```python
from build123d import *

# Parameters (mm, degrees)
HOLE_WIZARD_M3_1_D = 2.5


with BuildPart() as part:
    # 草图1 → 旋转1 (revolve)
    with BuildSketch(Plane.XY, mode=Mode.PRIVATE) as revolve_1_sk:
        Polygon((70, 0), (76.75, 0), (76.75, 3), (75, 3), (75, 11), (70, 11), align=None)
    revolve(revolve_1_sk.sketch.rotate(Axis((0, 51.694672702, 0), (0, -1, 0)), 90), axis=Axis((0, 51.694672702, 0), (0, -1, 0)))

    # M3 螺纹孔1 (through all)
    with Locations(Plane(origin=(0, 11, 0), x_dir=(1, 0, 0), z_dir=(0, 1, 0))):
        with Locations((-51.265241636, 51.265241636), (0, 72.5), (51.265241636, 51.265241636), (72.5, 0), (51.265241636, -51.265241636), (0, -72.5), (-51.265241636, -51.265241636), (-72.5, 0)):
            Hole(HOLE_WIZARD_M3_1_D / 2)


solid = part.part
```
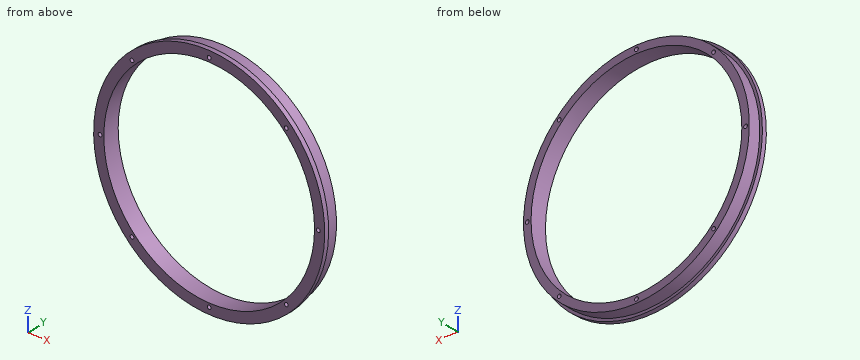
Part model, mm, in its own coordinate system. Coordinates: 2 decimals unless noted, no trailing zeros. Loops run counter-clockwise (first coordinate to the right, second up) from the corner with the lowest first, then second, coordinate; pieces in that order, holes last. Notation, with made-up numbers: (33.25, 87.25) - (52.25, 87.25) arc R24 cw to (52.25, 98.25) - close; hole circle Ø3 at (33, 82). An arc over 180 degrees is marked (long way). Write item = value, one per line. Start each with the question number.
Item 1: Cut at B-B, the plane z = 60. Give the cut face in (x, y).
Item 2: Wall check: L1, parallel to Z at x = 52, y = 5.5; L2, parallel to X at y = 2.75, z = 52; L3, parallel to X at y = 1.75, z = 18. Give the ranges that are in metal, low to high. Write a range as from..to.
Item 3: Flat gauge pins, fed straight in: pin 1 Ø2 at (x, z) = (72.5, 0) entering from +Y; pin 2 Ø2 at (x, y) = (-20.5, 6.5) entering from +Z; pin 3 Ø3 at (y, z) = (2.5, 11.5) entering from +X; pin 4 Ø2 at (y, z) = (5.5, -2.5) entering from +X (3 decimals). Where does each tip first touch, or does it go through?
Item 4: Cut at C-C, the plane y = 6. State how many separate pieces and enclosed holes the cut face has, and give its area (3 significant figures).
Item 5: Cut at A-A, the plane x = -46. Give the cut face in (y, z).
The answers:
q1.outline = (-47.86, 0) - (-36.06, 0) - (-36.06, 11) - (-45, 11) - (-45, 3) - (-47.86, 3) - close; (36.06, 0) - (47.86, 0) - (47.86, 3) - (45, 3) - (45, 11) - (36.06, 11) - close
q2.L1 = -54.05..-52.28, -50.25..-46.86, 46.86..50.25, 52.28..54.05
q2.L2 = -56.45..-52.28, -50.25..-46.86, 46.86..50.25, 52.28..56.45
q2.L3 = -74.61..-67.65, 67.65..74.61
q3.pin_1 = through
q3.pin_2 = 72.42
q3.pin_3 = 76.1
q3.pin_4 = 74.985
q4.separate_pieces = 1
q4.enclosed_holes = 9
q4.area = 2,240 mm2
q5.outline = (0, -61.44) - (3, -61.44) - (3, -59.24) - (11, -59.24) - (11, -52.76) - (0, -52.76) - close; (0, 52.76) - (11, 52.76) - (11, 59.24) - (3, 59.24) - (3, 61.44) - (0, 61.44) - close
